Design review of the part built by this model. Coordinates are the model's own, in mm. Face numbers are marked on the shaded views. A direction names the side the tool comes from. Round coordinates to 2 decimals unless told otherwise and drop trailing zeros. Write each loop counter-clockwise with the first axis right and the second up, starting at its lowest first coordinate (ties: lowest second). Pieces come first, ordered by that corner, then holes. Notation, with made-up numbers: M -1,71.25 L 30,71.25 A15 cw 30,96.25 Z; hole C 33,81.5 d9. An arc over 180 degrees is marked long. One line per question, with ' | ' between items. Start each with the question number.
Item 1: For L1, parallel to X at y = 14.5, z = -783; L2, parallel to X at y = 158, z = -750; L3, parallel to Y at x = -144.5, z = -777, list the stretches that pass through material, from the lowest coordinate up.
Item 2: Insertion check: pin 1 Ø1 at (y, z) = (79.5, -654.5) entering from +X; pin 2 Ø4 at (y, z) = (100.5, -655) entering from -X; pin 3 Ø5 at (y, z) = (107, -806.5) entering from +X. Each pin has a flat end and moves straight along its axis. Give the tip position at first contact, or say it passes through.
Item 3: Add section A-A, the plane z = -923. State the section outline as (x, y) points, and give its area (3 significant figures).
Item 4: Add section B-B, the plane y = 63.5. State the section outline as (x, z) points, and give its area (3 significant figures).
Item 5: Add section C-C, the plane x = -151.5. State the section outline as (y, z) points, and give its area (3 significant figures).
Item 6: Machinability: for the marked faces 1 and 2, which of the approach directions +Z, -Z, +X, -X, +Y, -Y give a long, thin tool a straight path to every point of the face, cutting with its end or side? Answer none if there is none.
```python
from build123d import *

# Parameters (mm, degrees)
SKETCH1_W               = 370
SKETCH1_H               = 370
BOSS_EXTRUDE1_DEPTH     = 1000
FILLET1_R               = 100
SHELL1_T                = -3
SKETCH2_W               = 241.73479806
SKETCH2_H               = 394.761154712
CUT_EXTRUDE1_DEPTH      = 2018.039910364
CUT_EXTRUDE2_DEPTH      = 1034.125839383
CUT_EXTRUDE2_DEPTH_BACK = 1034.125839383
SKETCH3_W               = 1896.128472869
SKETCH3_H               = 1300.286243779
SKETCH5_W               = 669.384629734
SKETCH5_H               = 44.432040192
SKETCH5_H_2             = 62.844566938
CUT_EXTRUDE4_DEPTH      = 1034.658550973
SKETCH4_W               = 536.60110681
SKETCH4_H               = 206.247567531
CUT_EXTRUDE5_DEPTH      = 1018.539609917


with BuildPart() as part:
    # Sketch1 → Boss-Extrude1 (new, symmetric)
    with BuildSketch(Plane.XY):
        Rectangle(SKETCH1_W, SKETCH1_H)
    extrude(amount=BOSS_EXTRUDE1_DEPTH, both=True)

    # Fillet1
    fillet1_edges = [part.edges().sort_by_distance(p)[0] for p in [
        (-185, 185, 0),
        (185, 185, 0),
        (185, -185, 0),
        (-185, -185, 0),
    ]]
    fillet(fillet1_edges, radius=FILLET1_R)

    # Shell1
    shell1_openings = [part.faces().sort_by_distance(p)[0] for p in [
        (0, 0, -1000),
    ]]
    offset(amount=SHELL1_T, openings=shell1_openings, kind=Kind.INTERSECTION)

    # Sketch2 → Cut-Extrude1 (cut, through all)
    with BuildSketch(Plane.XY.offset(1000)):
        with Locations((120.86739903, -12.380577356)):
            Rectangle(SKETCH2_W, SKETCH2_H)
    extrude(amount=-CUT_EXTRUDE1_DEPTH, mode=Mode.SUBTRACT)

    # Sketch3 → Cut-Extrude2 (cut, two sides: drawn at the far end of the back side and taken through both)
    with BuildSketch(Plane(origin=(-182, 0, 0), x_dir=(0, 0, -1), z_dir=(1, 0, 0)).offset(-CUT_EXTRUDE2_DEPTH_BACK)):
        with Locations((-400.064236435, -68.17726838)):
            Rectangle(SKETCH3_W, SKETCH3_H)
    extrude(amount=CUT_EXTRUDE2_DEPTH + CUT_EXTRUDE2_DEPTH_BACK, mode=Mode.SUBTRACT)

    # Sketch5 → Cut-Extrude4 (cut, through all)
    with BuildSketch(Plane.ZY.offset(185)):
        with Locations((-762.41238843, 198.216020096)):
            Rectangle(SKETCH5_W, SKETCH5_H)
        with Locations((-762.41238843, -207.422283469)):
            Rectangle(SKETCH5_W, SKETCH5_H_2)
    extrude(amount=-CUT_EXTRUDE4_DEPTH, mode=Mode.SUBTRACT)

    # Sketch4 → Cut-Extrude5 (cut, through all)
    with BuildSketch(Plane.ZY.offset(185)):
        with Locations((-731.699446595, -103.123783766)):
            Rectangle(SKETCH4_W, SKETCH4_H)
    extrude(amount=-CUT_EXTRUDE5_DEPTH, mode=Mode.SUBTRACT)


solid = part.part
```
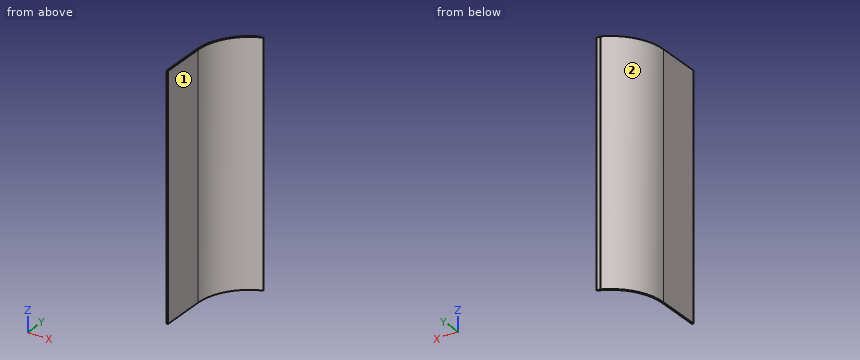
Computed values:
1) L1: x = -185 to -182 | L2: x = -153.34 to -148.87 | L3: y = 161.61 to 165.37
2) pin 1: stops at x = -182 | pin 2: stops at x = -184.08 | pin 3: stops at x = -178.85
3) outline: M -185,0 L -182,0 L -182,85 A97 cw -118.59,176 L -126.46,176 A100 ccw -185,85 Z | area: 603 mm^2
4) outline: M -185,-1000 L -182,-1000 L -182,-548 L -185,-548 Z | area: 1,360 mm^2
5) outline: M 155.62,-1000 L 159.68,-1000 L 159.68,-548 L 155.62,-548 Z | area: 1,840 mm^2
6) face 1: +Z, -Z, +X, -Y | face 2: +Z, -Z, -X, +Y
